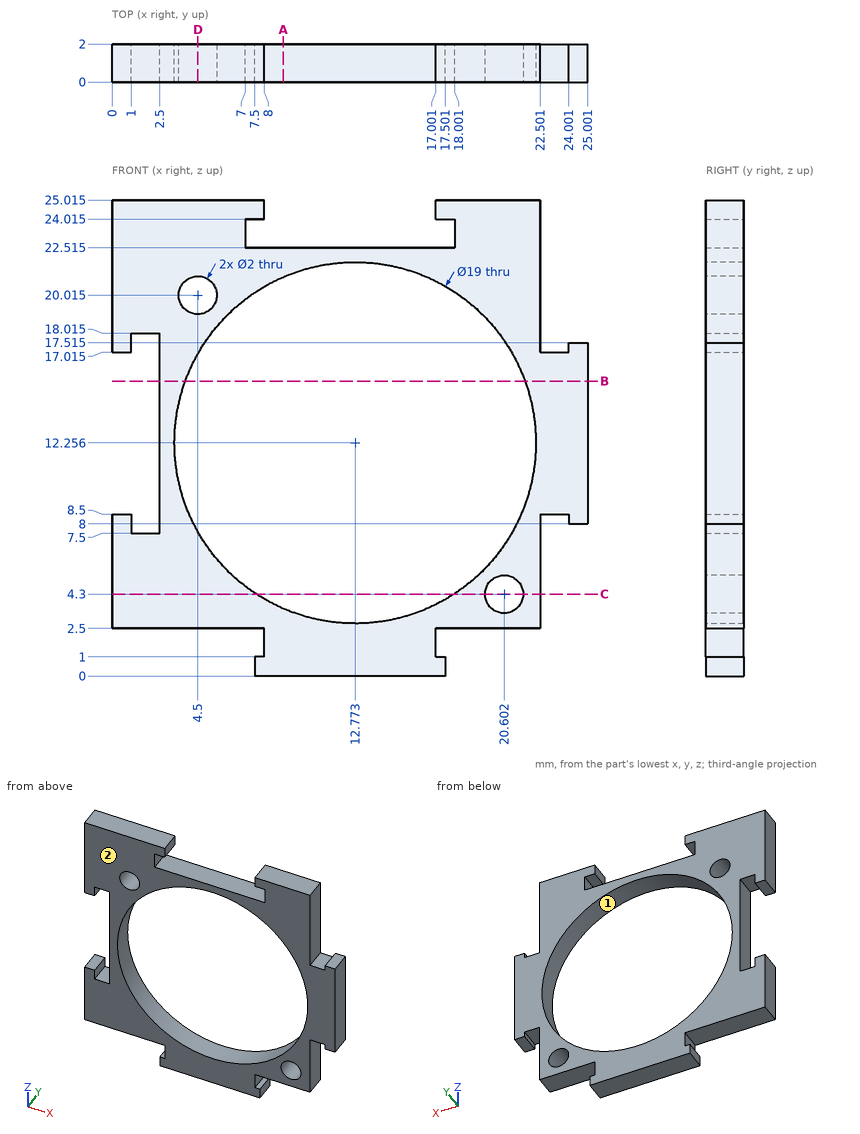
Here's the drawing with two shaded views (mm, measured from the low corner). I have some questions. Coordinates: 2 decimals unless noted, no trailing zeros. Loops run counter-clockwise (first coordinate to the right, second up) from the corner with the lowest first, then second, coordinate; pieces in that order, holes last. Notation, with made-up numbers: (36.25, -36) -> (77.25, -36) arc R16 ccw to (77.25, -28) -> close; hole circle Ø1 at (-14, 1). An arc over 180 degrees is marked (long way). Answer in a Markdown table with one row per item.
(1) Will these pins go through, and if not, where does the flat tip stop? pin 1 Ø0.8 at (x, y) = (23, 1) entering from -Z; pin 2 Ø0.5 at (y, z) = (1, 0.5) entering from +X; pin 3 Ø1.1 at (x, y) = (24.5, 1.5) entering from -Z.
Results found:
| item | result |
|---|---|
| pin 1 | stops at z = 8.5 |
| pin 2 | stops at x = 17.5 |
| pin 3 | stops at z = 8 |
(2) Imagine slicing it at A-A (x = 9). List the corners of the cut face in (y, z) for me (1 decimal).
Results found:
| item | result |
|---|---|
| outline | (0, 0) -> (2, 0) -> (2, 3.5) -> (0, 3.5) -> close; (0, 21) -> (2, 21) -> (2, 22.5) -> (0, 22.5) -> close |
(3) Imagine slicing it at C-C (z = 4.3). List the corners of the cut face in (x, y) for me (1 decimal).
Results found:
| item | result |
|---|---|
| outline | (0, 0) -> (7.6, 0) -> (7.6, 2) -> (0, 2) -> close; (18, 0) -> (19.6, 0) -> (19.6, 2) -> (18, 2) -> close; (21.6, 0) -> (22.5, 0) -> (22.5, 2) -> (21.6, 2) -> close |
(4) Thinking about a two-plate mould opening in X: for the marked faces 1 and 2, which applies, released by +X, released by -X, zero draft, split by the parting line, or undercut?
Results found:
| item | result |
|---|---|
| face 1 | undercut |
| face 2 | zero draft |
(5) Imagine slicing it at D-D (x = 4.5). List the corners of the cut face in (y, z) for me (1 decimal).
Results found:
| item | result |
|---|---|
| outline | (0, 2.5) -> (2, 2.5) -> (2, 7.6) -> (0, 7.6) -> close; (0, 16.9) -> (2, 16.9) -> (2, 19) -> (0, 19) -> close; (0, 21) -> (2, 21) -> (2, 25) -> (0, 25) -> close |
(6) Imagine slicing it at B-B (z = 15.5). List the corners of the cut face in (x, y) for me (1 decimal).
Results found:
| item | result |
|---|---|
| outline | (2.5, 0) -> (3.8, 0) -> (3.8, 2) -> (2.5, 2) -> close; (21.7, 0) -> (25, 0) -> (25, 2) -> (21.7, 2) -> close |
(7) If I drill on probe 1 along Z at (x, y) = (20.5, 1.8) (1 decimal); probe 2 along Z at (x, y) = (4.5, 0.95) (1 decimal); probe 3 along X at (y, z) = (0.7, 18.25) (1 decimal), over which ranges is the centre line in solid material (lowest first)?
Results found:
| item | result |
|---|---|
| probe 1 | z = 2.5 to 3.3, 5.3 to 6.7, 17.8 to 25 |
| probe 2 | z = 2.5 to 7.6, 16.9 to 19, 21 to 25 |
| probe 3 | x = 0 to 5.4, 20.1 to 22.5 |
